CAD build for the part. Positions are in the model's coordinates, mm. Round coordinates to 2 decimals unless told otherwise and drop trailing zeros. Loops run counter-clockwise (first coordinate to the right, second up) from the corner with the lowest first, then second, coordinate; pieces in that order, holes last.
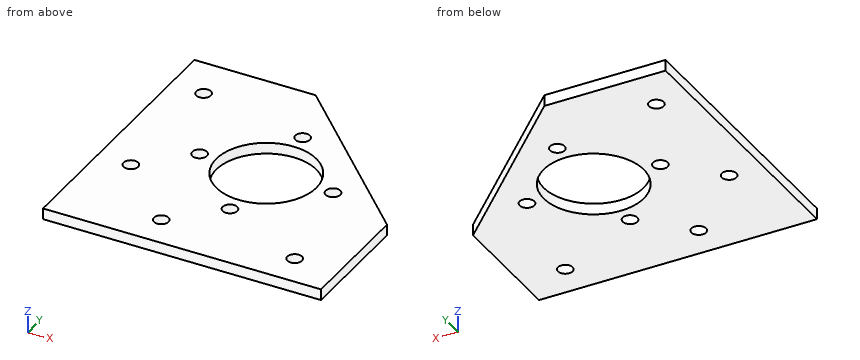
from build123d import *

# Parameters (mm, degrees)
SKETCH_1_R            = 22.5
EXTRUDE_1_DEPTH       = 5
HOLE_WIZARD_M61_D     = 6.6
HOLE_WIZARD_M61_DEPTH = 10
HOLE_WIZARD_M61_TIP   = 1.982840043


with BuildPart() as part:
    # Эскиз1 → Бобышка-Вытянуть1 (new body)
    with BuildSketch(Plane.XY):
        Polygon((0, 0), (0, 125), (54.497474683, 125), (125, 54.497474683), (125, 0), align=None)
        with Locations((65, 65)):
            Circle(SKETCH_1_R, mode=Mode.SUBTRACT)
    extrude(amount=EXTRUDE_1_DEPTH)

    # Отверстие с зазором M61
    with Locations(Plane(origin=(0, 0, 0), x_dir=(-1, 0, 0), z_dir=(0, 0, -1))):
        with Locations((-95, 65), (-65, 95), (-35, 65), (-65, 35), (-105, 15), (-45, 15), (-15, 45), (-15, 105)):
            Hole(HOLE_WIZARD_M61_D / 2, depth=HOLE_WIZARD_M61_DEPTH)
            with Locations((0, 0, -(HOLE_WIZARD_M61_DEPTH + HOLE_WIZARD_M61_TIP / 2))):  # 118° drill point
                Cone(0, HOLE_WIZARD_M61_D / 2, HOLE_WIZARD_M61_TIP, mode=Mode.SUBTRACT)


solid = part.part
Item 1: Flat gauge pins, fed straight in: P1, Ø2, axis at x = 100.5, z = 2, coming from the -Y side; P2, Ø1, axis at y = 60, z = 2.5, coming from the +X side. Where does each tip first touch, or does it go through?
Verdict:
P1: stops at y = 0
P2: stops at x = 120
Item 2: Cut at A-A (y = 15). List the corners of the cut face in (x, z), plus the area to 3 significant figures.
Verdict:
outline: (0, 0) - (41.7, 0) - (41.7, 5) - (0, 5) - close; (48.3, 0) - (101.7, 0) - (101.7, 5) - (48.3, 5) - close; (108.3, 0) - (125, 0) - (125, 5) - (108.3, 5) - close
area: 559 mm2
Item 3: Wall check: L1, parallel to Y at x = 15, z = 1.6; L2, parallel to X at y = 46, z = 1.7; L3, parallel to X at y = 77, z = 0.5. Give the ranges that are in metal, low to high.
Verdict:
L1: y = 0 to 41.7, 48.3 to 101.7, 108.3 to 125
L2: x = 0 to 11.86, 18.14 to 52.95, 77.05 to 125
L3: x = 0 to 45.97, 84.03 to 102.5
Item 4: Cut at C-C (z = 1). State how many separate pieces and enclosed holes the cut face has, plus the area to 3 significant figures.
Verdict:
separate pieces: 1
enclosed holes: 9
area: 11,300 mm2
Item 5: Cut at D-D (x = 105). List the corners of the cut face in (y, z).
Verdict:
outline: (0, 0) - (11.7, 0) - (11.7, 5) - (0, 5) - close; (18.3, 0) - (74.5, 0) - (74.5, 5) - (18.3, 5) - close
